Work out the finished part from the listing and answer in its coordinate system (mm). A direction names the side the tool comes from. Round coordinates to 2 decimals unless told otherwise and drop trailing zeros. Order: outer loops, then holes, each group sorted by start corner. A loop starts at its lowest first (then second) coordinate and runs counter-clockwise, first axis right, second up. Notation, with made-up numbers: (84, 24) -> (128, 24) arc R17 cw to (128, 42) -> close; hole circle Ø1 at (-36.5, 22.5). An arc over 180 degrees is marked (long way). Use one line per item in the form item = value.
```python
from build123d import *

# Parameters (mm, degrees)
BOSS_EXTRUDE2_DEPTH = 40
SKETCH6_R           = 3.25
SKETCH6_R_2         = 1.7
CUT_EXTRUDE1_DEPTH  = 72.582120673
SKETCH7_R           = 1.7
CUT_EXTRUDE2_DEPTH  = 58.818545186


with BuildPart() as part:
    # Sketch3 → Boss-Extrude2 (new body)
    with BuildSketch(Plane(origin=(0, 0, 0), x_dir=(0, 0, -1), z_dir=(1, 0, 0))):
        with BuildLine():
            Line((0, -23.186119874), (50, -23.186119874))
            Line((50, -23.186119874), (50, -5.186119874))
            Line((50, -5.186119874), (20, -5.186119874))
            ThreePointArc((20, -5.186119874), (18.585786438, -4.600333436), (18, -3.186119874))
            Line((18, -3.186119874), (18, 26.813880126))
            Line((18, 26.813880126), (0, 26.813880126))
            Line((0, 26.813880126), (0, -23.186119874))
        make_face()
    extrude(amount=BOSS_EXTRUDE2_DEPTH)

    # Sketch6 → Cut-Extrude1 (cut, through all)
    with BuildSketch(Plane(origin=(0, -5.186119874, 0), x_dir=(1, 0, 0), z_dir=(0, 1, 0))):
        with Locations(Location((20, 33, 0), (0, 0, 270))):
            Circle(SKETCH6_R)
        with Locations(Location((9, 33, 0), (0, 0, 270))):
            Circle(SKETCH6_R_2)
        with Locations(Location((20, 44, 0), (0, 0, 270))):
            Circle(SKETCH6_R_2)
        with Locations(Location((31, 33, 0), (0, 0, 270))):
            Circle(SKETCH6_R_2)
        with Locations(Location((20, 22, 0), (0, 0, 270))):
            Circle(SKETCH6_R_2)
    extrude(amount=-CUT_EXTRUDE1_DEPTH, mode=Mode.SUBTRACT)

    # Sketch7 → Cut-Extrude2 (cut, through all)
    with BuildSketch(Plane(origin=(0, 0, -18), x_dir=(-1, 0, 0), z_dir=(0, 0, -1))):
        with Locations(Location((-30, 20, 0), (0, 0, 90))):
            Circle(SKETCH7_R)
        with Locations(Location((-10, 20, 0), (0, 0, 90))):
            Circle(SKETCH7_R)
        with Locations(Location((-30, 5, 0), (0, 0, 90))):
            Circle(SKETCH7_R)
        with Locations(Location((-10, 5, 0), (0, 0, 90))):
            Circle(SKETCH7_R)
    extrude(amount=-CUT_EXTRUDE2_DEPTH, mode=Mode.SUBTRACT)


solid = part.part
```
Item 1: The part is cut by section B-B, the plane y = -6.5. Give the vertices of the cut face in (x, z), and give its area (3 significant figures).
Findings:
outline = (0, -50) -> (40, -50) -> (40, 0) -> (0, 0) -> close; hole circle Ø3.4 at (9, -33); hole circle Ø6.5 at (20, -33); hole circle Ø3.4 at (20, -44); hole circle Ø3.4 at (20, -22); hole circle Ø3.4 at (31, -33)
area = 1,930 mm^2
Item 2: For faces 1 (the flat face through (20, 12, -18)), 2 (the flat face through (0, -9, -19)), determine the directions among +Z, -Z, +X, -X, +Y, -Y from which every point of the face is accessible in a straight line to the end or side of a thin tool.
Findings:
face_1 = -Z, +X, -X, +Y
face_2 = +Z, -Z, -X, +Y, -Y
Item 3: The part is cut by section D-D, the plane z = -33. Give the vertices of the cut face in (x, y), and give its area (3 significant figures).
Findings:
outline = (0, -23.19) -> (7.3, -23.19) -> (7.3, -5.19) -> (0, -5.19) -> close; (10.7, -23.19) -> (16.75, -23.19) -> (16.75, -5.19) -> (10.7, -5.19) -> close; (23.25, -23.19) -> (29.3, -23.19) -> (29.3, -5.19) -> (23.25, -5.19) -> close; (32.7, -23.19) -> (40, -23.19) -> (40, -5.19) -> (32.7, -5.19) -> close
area = 481 mm^2
Item 4: The part is cut by section C-C, the plane z = -44. Give the vertices of the cut face in (x, y).
Findings:
outline = (0, -23.19) -> (18.3, -23.19) -> (18.3, -5.19) -> (0, -5.19) -> close; (21.7, -23.19) -> (40, -23.19) -> (40, -5.19) -> (21.7, -5.19) -> close
Item 5: Determine the mould class of faces 3 (the cylindrical face through (29.5, -14.1, -32.2)), 4 (the flat face through (20, -23.186, -25)), 5 (the flat face through (20, 2, 0)), 6 (the cylindrical face through (21.15, -14.06, -45.25)) for opening direction Z: released by +Z, released by -Z, zero draft, split by the parting line, or undercut.
Findings:
face_3 = undercut
face_4 = zero draft
face_5 = released by +Z
face_6 = undercut
Item 6: Consider line 1 along X through (y, z) = (5, -4); line 2 along X through (y, z) = (-12.5, -44); line 3 along X through (y, z) = (-17.75, -33). Determine where each line is inside the solid, lowest interval first.
Findings:
line_1 = 0 to 8.3, 11.7 to 28.3, 31.7 to 40
line_2 = 0 to 18.3, 21.7 to 40
line_3 = 0 to 7.3, 10.7 to 16.75, 23.25 to 29.3, 32.7 to 40
Item 7: Flat-ended cylindrical pins translate along their axes: P1, Ø5.5, axis at x = 20, z = -22, coming from the -Y side; P2, Ø2, axis at x = 23, z = -29.5, coming from the +Y side; P3, Ø1.5, axis at x = 24, y = 13.5, coming from the -Z side. Find the tip coordinate at first contact, or state that the pin passes through.
Findings:
P1 = -23.19
P2 = -5.19
P3 = -18
Item 8: The part is cut by section A-A, the plane x = 20. Give the vertices of the cut face in (y, z), and give its area (3 significant figures).
Findings:
outline = (-23.19, -50) -> (-5.19, -50) -> (-5.19, -45.7) -> (-23.19, -45.7) -> close; (-23.19, -42.3) -> (-5.19, -42.3) -> (-5.19, -36.25) -> (-23.19, -36.25) -> close; (-23.19, -29.75) -> (-5.19, -29.75) -> (-5.19, -23.7) -> (-23.19, -23.7) -> close; (-23.19, -20.3) -> (-5.19, -20.3) -> (-5.19, -20) arc R2 cw to (-3.19, -18) -> (26.81, -18) -> (26.81, 0) -> (-23.19, 0) -> close
area = 1,240 mm^2
